from build123d import *

# Parameters (mm, degrees)
SKETCH_1_R      = 10.5
SKETCH_1_R_2    = 7.5
SKETCH_1_R_3    = 2
SKETCH_1_R_4    = 2.1
EXTRUDE_1_DEPTH = 4


with BuildPart() as part:
    # 草图1 → 凸台-拉伸1 (new body)
    with BuildSketch(Plane(origin=(0, 0, 0), x_dir=(1, 0, 0), z_dir=(0, 1, 0))):
        with BuildLine():
            Line((0, 10), (0, 0))
            Line((0, 0), (60, 0))
            Line((60, 0), (60, 10))
            Line((60, 10), (56.095182285, 18.373908614))
            Line((56.095182285, 18.373908614), (55.431150168, 19.5))
            ThreePointArc((55.431150168, 19.5), (55.079606541, 21.641551662), (56.264363658, 23.459841248))
            ThreePointArc((56.264363658, 23.459841248), (70.812010618, 78.957314928), (19.020417199, 103.639990393))
            ThreePointArc((19.020417199, 103.639990393), (16.99979992, 103.840191523), (15.569521651, 105.281468301))
            Line((15.569521651, 105.281468301), (9.668235965, 117.936816295))
            ThreePointArc((9.668235965, 117.936816295), (-13.775496492, 127.647528231), (-25.492512153, 105.139350566))
            Line((-25.492512153, 105.139350566), (0, 10))
        make_face()
        with Locations(Location((-7.352321507, 110, 0), (0, 0, 270))):
            Circle(SKETCH_1_R, mode=Mode.SUBTRACT)
        with Locations(Location((30, 60, 0), (0, 0, 270))):
            Circle(SKETCH_1_R_2, mode=Mode.SUBTRACT)
        with Locations(Location((30, 80, 0), (0, 0, 270))):
            Circle(SKETCH_1_R_3, mode=Mode.SUBTRACT)
        with Locations(Location((47.320508076, 50, 0), (0, 0, 270))):
            Circle(SKETCH_1_R_3, mode=Mode.SUBTRACT)
        with Locations(Location((12.679491924, 50, 0), (0, 0, 270))):
            Circle(SKETCH_1_R_3, mode=Mode.SUBTRACT)
        with Locations(Location((23, 5, 0), (0, 0, 270))):
            Circle(SKETCH_1_R_4, mode=Mode.SUBTRACT)
        with Locations(Location((9, 5, 0), (0, 0, 270))):
            Circle(SKETCH_1_R_4, mode=Mode.SUBTRACT)
        with Locations(Location((37, 5, 0), (0, 0, 90))):
            Circle(SKETCH_1_R_4, mode=Mode.SUBTRACT)
        with Locations(Location((51, 5, 0), (0, 0, 90))):
            Circle(SKETCH_1_R_4, mode=Mode.SUBTRACT)
        with BuildLine():
            Line((26.5, 20.5), (31.5, 20.5))
            ThreePointArc((31.5, 20.5), (32.5, 19.5), (31.5, 18.5))
            Line((31.5, 18.5), (26.5, 18.5))
            ThreePointArc((26.5, 18.5), (25.5, 19.5), (26.5, 20.5))
        make_face(mode=Mode.SUBTRACT)
        with BuildLine():
            Line((-0.975772037, 35.443910191), (2.27680142, 31.646441837))
            ThreePointArc((2.27680142, 31.646441837), (2.167822441, 30.236433474), (0.757814079, 30.345412454))
            Line((0.757814079, 30.345412454), (-2.494759379, 34.142880808))
            ThreePointArc((-2.494759379, 34.142880808), (-2.3857804, 35.552889171), (-0.975772037, 35.443910191))
        make_face(mode=Mode.SUBTRACT)
        with BuildLine():
            Line((60.975772037, 35.443910191), (57.72319858, 31.646441837))
            ThreePointArc((57.72319858, 31.646441837), (57.832177559, 30.236433474), (59.242185921, 30.345412454))
            Line((59.242185921, 30.345412454), (62.494759379, 34.142880808))
            ThreePointArc((62.494759379, 34.142880808), (62.3857804, 35.552889171), (60.975772037, 35.443910191))
        make_face(mode=Mode.SUBTRACT)
    extrude(amount=EXTRUDE_1_DEPTH)


solid = part.part
Read the model definition and answer for the solid it produces. Units are mm, in the model's axes. A direction names the side the tool comes from. Coordinates: 2 decimals unless noted, no trailing zeros. Order: outer loops, then holes, each group sorted by start corner. A loop starts at its lowest first (then second) coordinate and runs counter-clockwise, first axis right, second up. Notation, with made-up numbers: M -33,14.5 L 16,14.5 A9 ccw 16,23.5 Z; hole C -6,88 d5. An arc over 180 degrees is marked long. Put each result on its own line as item: value. Start each with the question number.
Item 1: Given pin 1 Ø2.5 at (x, z) = (12.68, -50) entering from -Y; pin 2 Ø1.5 at (x, y) = (-5, 1) entering from -Z; pin 3 Ø1.2 at (x, y) = (30, 1.5) entering from -Z; pin 4 Ø1 at (y, z) = (0.5, -104) entering from -X, each flat-ended and moving along its own axis, determine where each tip first touches the part or whether it passes through.
Item 2: Section C-C, the plane x = -16.5 is taken. Determine the outline of the cut face in (y, z).
Item 3: Section B-B, the plane z = -60 is taken. Determine the outline of the cut face in (x, y), plus the area to 3 significant figures.
Item 4: Section A-A, the plane x = 30 is taken. Determine the outline of the cut face in (y, z).
Item 5: Consider probe 1 along X at (y, z) = (2, -5); probe 2 along X at (y, z) = (2.5, -32.5); probe 3 along X at (y, z) = (0.9, -50). Determine where each line is inside the solid, lowest interval first. Write a range as [from, to].
Item 6: For faces 4 (the face through (58.075, 1.972, -14.128)), 5 (the face through (59.37, 1.97, -33.57)), 6 (the face through (24, 4, -65)), determine the directions among +Z, -Z, +X, -X, +Y, -Y from which every point of the face is accessible in a straight line to the end or side of a thin tool.
Item 7: Section D-D, the plane y = 2.45 is taken. Count the separate pieces of the cut face and the enclosed holes in it, plus the area to 3 significant figures.
Item 8: The mould has two halves that part along Z. Classify faces 1 (the face through (29, 2, -18.5)), 2 (the face through (24, 0, -65)), 3 (the face through (12.66, 1.97, -111.52)): +Z half, -Z half, draft (parallel to the pull), parting line (faces both ways), or undercut.
Computed:
1. pin 1: passes through
1. pin 2: stops at z = -128.71
1. pin 3: stops at z = -105
1. pin 4: stops at x = -25.32
2. outline: M 0,-126.4 L 4,-126.4 L 4,-115.15 L 0,-115.15 Z; M 0,-104.85 L 4,-104.85 L 4,-71.58 L 0,-71.58 Z
3. outline: M -13.4,0 L 22.5,0 L 22.5,4 L -13.4,4 Z; M 37.5,0 L 75,0 L 75,4 L 37.5,4 Z
3. area: 294 mm2
4. outline: M 0,-105 L 4,-105 L 4,-82 L 0,-82 Z; M 0,-78 L 4,-78 L 4,-67.5 L 0,-67.5 Z; M 0,-52.5 L 4,-52.5 L 4,-20.5 L 0,-20.5 Z; M 0,-18.5 L 4,-18.5 L 4,0 L 0,0 Z
5. probe 1: x = [0, 6.9], [11.1, 20.9], [25.1, 34.9], [39.1, 48.9], [53.1, 60]
5. probe 2: x = [-6.03, -1.09], [1.55, 58.45], [61.09, 65.62]
5. probe 3: x = [-10.72, 10.68], [14.68, 45.32], [49.32, 73.87]
6. face 4: +X, +Y, -Y
6. face 5: +Y, -Y
6. face 6: +Z, -Z, +X, -X, +Y
7. separate pieces: 1
7. enclosed holes: 12
7. area: 8,150 mm2
8. face 1: undercut
8. face 2: draft
8. face 3: -Z half
